Can you work these out from the model? Positions are in its coordinate system, mm. Face numbers are marked on the shaded views. A direction names the side the tool comes from. Coordinates: 2 decimals unless noted, no trailing zeros. Order: outer loops, then holes, each group sorted by start corner. A loop starts at its lowest first (then second) coordinate and runs counter-clockwise, first axis right, second up. Notation, with made-up numbers: (-36.75, 63) -> (20.25, 63) arc R27 cw to (20.25, 79) -> close; hole circle Ø7 at (19, 32). An arc over 180 degrees is marked (long way). Write item = value, one per line.
```python
from build123d import *

# Parameters (mm, degrees)
SKETCH_1_W          = 179
SKETCH_1_H          = 182
EXTRUDE_1_DEPTH     = 15
SKETCH_2_R          = 15
CUT_EXTRUDE_1_DEPTH = 129.51556326
CUT_EXTRUDE_3_DEPTH = 129.51556326
FILLET_1_R          = 20
EXTRUDE_2_DEPTH     = 90
FILLET_2_R          = 15
EXTRUDE_3_DEPTH     = 5
SKETCH_7_W          = 172
SKETCH_7_H          = 155
EXTRUDE_4_DEPTH     = 15
CUT_EXTRUDE_4_DEPTH = 15
FILLET_3_R          = 48
SKETCH_9_R          = 4.5
CUT_EXTRUDE_5_DEPTH = 15
SKETCH_11_W         = 69
SKETCH_11_H         = 3
EXTRUDE_5_DEPTH     = 18
FILLET_4_R          = 18
SKETCH_12_R         = 12
CUT_EXTRUDE_6_DEPTH = 12
SKETCH_13_R         = 11
CUT_EXTRUDE_7_DEPTH = 6
FILLET_5_R          = 2


with BuildPart() as part:
    # 草图1 → 凸台-拉伸1 (new body)
    with BuildSketch(Plane(origin=(0, 0, 0), x_dir=(1, 0, 0), z_dir=(0, 1, 0))):
        Rectangle(SKETCH_1_W, SKETCH_1_H)
    extrude(amount=EXTRUDE_1_DEPTH)

    # 草图2 → 切除-拉伸1 (cut, through all)
    with BuildSketch(Plane(origin=(0, 15, 0), x_dir=(1, 0, 0), z_dir=(0, 1, 0))):
        with Locations(Location((0, 22, 0), (0, 0, 270))):
            Circle(SKETCH_2_R)
    extrude(amount=-CUT_EXTRUDE_1_DEPTH, mode=Mode.SUBTRACT)

    # 草图4 → 切除-拉伸3 (cut, through all)
    with BuildSketch(Plane(origin=(0, 15, 0), x_dir=(1, 0, 0), z_dir=(0, 1, 0))):
        with BuildLine():
            Line((-77, -72.5), (-73, -72.5))
            ThreePointArc((-73, -72.5), (-67.5, -78), (-73, -83.5))
            Line((-73, -83.5), (-77, -83.5))
            ThreePointArc((-77, -83.5), (-82.5, -78), (-77, -72.5))
        make_face()
        with BuildLine():
            Line((-77, -22.5), (-73, -22.5))
            ThreePointArc((-73, -22.5), (-67.5, -28), (-73, -33.5))
            Line((-73, -33.5), (-77, -33.5))
            ThreePointArc((-77, -33.5), (-82.5, -28), (-77, -22.5))
        make_face()
        with BuildLine():
            Line((-77, 7.5), (-73, 7.5))
            ThreePointArc((-73, 7.5), (-67.5, 2), (-73, -3.5))
            Line((-73, -3.5), (-77, -3.5))
            ThreePointArc((-77, -3.5), (-82.5, 2), (-77, 7.5))
        make_face()
        with BuildLine():
            Line((77, 7.5), (73, 7.5))
            ThreePointArc((73, 7.5), (67.5, 2), (73, -3.5))
            Line((73, -3.5), (77, -3.5))
            ThreePointArc((77, -3.5), (82.5, 2), (77, 7.5))
        make_face()
        with BuildLine():
            Line((77, -22.5), (73, -22.5))
            ThreePointArc((73, -22.5), (67.5, -28), (73, -33.5))
            Line((73, -33.5), (77, -33.5))
            ThreePointArc((77, -33.5), (82.5, -28), (77, -22.5))
        make_face()
        with BuildLine():
            Line((77, -72.5), (73, -72.5))
            ThreePointArc((73, -72.5), (67.5, -78), (73, -83.5))
            Line((73, -83.5), (77, -83.5))
            ThreePointArc((77, -83.5), (82.5, -78), (77, -72.5))
        make_face()
    extrude(amount=-CUT_EXTRUDE_3_DEPTH, mode=Mode.SUBTRACT)

    # 圆角1
    fillet_1_edges = [part.edges().sort_by_distance(p)[0] for p in [
        (89.5, 7.5, 91),
        (-89.5, 7.5, 91),
    ]]
    fillet(fillet_1_edges, radius=FILLET_1_R)

    # 草图5 → 凸台-拉伸2 (add)
    with BuildSketch(Plane(origin=(0, 15, 0), x_dir=(1, 0, 0), z_dir=(0, 1, 0))):
        Polygon((-64, 91), (-64, -45), (64, -45), (64, 91), (39, 91), (39, -29), (-39, -29), (-39, 91), align=None)
    extrude(amount=EXTRUDE_2_DEPTH)

    # 圆角2
    fillet_2_edges = [part.edges().sort_by_distance(p)[0] for p in [
        (-64, 60, 45),
        (64, 60, 45),
    ]]
    fillet(fillet_2_edges, radius=FILLET_2_R)

    # 草图6 → 凸台-拉伸3 (add, symmetric)
    with BuildSketch(Plane(origin=(0, 0, 0), x_dir=(0, 0, -1), z_dir=(1, 0, 0))):
        with BuildLine():
            Line((-45, 105), (-60, 105))
            Line((-60, 105), (-49, 80))
            Line((-49, 80), (-49, 54.937451095))
            ThreePointArc((-49, 54.937451095), (-57.014709064, 30.259525737), (-78, 15))
            Line((-78, 15), (-45, 15))
            Line((-45, 15), (-45, 105))
        make_face()
    extrude(amount=EXTRUDE_3_DEPTH, both=True)

    # 草图7 → 凸台-拉伸4 (add)
    with BuildSketch(Plane(origin=(0, 105, 0), x_dir=(1, 0, 0), z_dir=(0, 1, 0))):
        with Locations((0, 13.5)):
            Rectangle(SKETCH_7_W, SKETCH_7_H)
    extrude(amount=EXTRUDE_4_DEPTH)

    # 草图8 → 切除-拉伸4 (cut)
    with BuildSketch(Plane(origin=(0, 120, 0), x_dir=(1, 0, 0), z_dir=(0, 1, 0))):
        Polygon((-86, 91), (-86, 60), (-64, 91), align=None)
        Polygon((64, 91), (86, 91), (86, 60), align=None)
    extrude(amount=-CUT_EXTRUDE_4_DEPTH, mode=Mode.SUBTRACT)

    # 圆角3
    fillet_3_edges = [part.edges().sort_by_distance(p)[0] for p in [
        (-86, 112.5, 64),
        (86, 112.5, 64),
    ]]
    fillet(fillet_3_edges, radius=FILLET_3_R)

    # 草图9 → 切除-拉伸5 (cut)
    with BuildSketch(Plane(origin=(0, 120, 0), x_dir=(1, 0, 0), z_dir=(0, 1, 0))):
        with Locations(Location((-72, 60, 0), (0, 0, 270))):
            Circle(SKETCH_9_R)
        with Locations(Location((-72, -16, 0), (0, 0, 270))):
            Circle(SKETCH_9_R)
        with Locations(Location((72, -16, 0), (0, 0, 270))):
            Circle(SKETCH_9_R)
        with Locations(Location((72, 60, 0), (0, 0, 270))):
            Circle(SKETCH_9_R)
    extrude(amount=-CUT_EXTRUDE_5_DEPTH, mode=Mode.SUBTRACT)

    # 草图11 → 凸台-拉伸5 (add, symmetric)
    with BuildSketch(Plane(origin=(0, 0, 0), x_dir=(0, 0, -1), z_dir=(1, 0, 0))):
        with Locations((5.5, 103.5)):
            Rectangle(SKETCH_11_W, SKETCH_11_H)
    extrude(amount=EXTRUDE_5_DEPTH, both=True)

    # 圆角4
    fillet_4_edges = [part.edges().sort_by_distance(p)[0] for p in [
        (-18, 103.5, -40),
        (18, 103.5, -40),
    ]]
    fillet(fillet_4_edges, radius=FILLET_4_R - 0.0001)  # a hair under: the kernel refuses the full size

    # 草图12 → 切除-拉伸6 (cut)
    with BuildSketch(Plane(origin=(0, 120, 0), x_dir=(1, 0, 0), z_dir=(0, 1, 0))):
        with Locations(Location((0, 22, 0), (0, 0, 270))):
            Circle(SKETCH_12_R)
    extrude(amount=-CUT_EXTRUDE_6_DEPTH, mode=Mode.SUBTRACT)

    # 草图13 → 切除-拉伸7 (cut)
    with BuildSketch(Plane(origin=(0, 108, 0), x_dir=(1, 0, 0), z_dir=(0, 1, 0))):
        with Locations(Location((0, 22, 0), (0, 0, 270))):
            Circle(SKETCH_13_R)
    extrude(amount=-CUT_EXTRUDE_7_DEPTH, mode=Mode.SUBTRACT)

    # 圆角5
    fillet_5_edges = [part.edges().sort_by_distance(p)[0] for p in [
        (-64, 15, -30.5),
        (64, 15, -30.5),
        (-27, 15, 45),
        (59.606601718, 15, 40.606601718),
        (-59.606601718, 15, 40.606601718),
        (27, 15, 45),
        (-5, 60, 45),
        (-5, 105, 52.5),
        (-5, 15, 61.5),
        (5, 60, 45),
        (5, 105, 52.5),
        (5, 15, 61.5),
    ]]
    fillet(fillet_5_edges, radius=FILLET_5_R)


solid = part.part
```
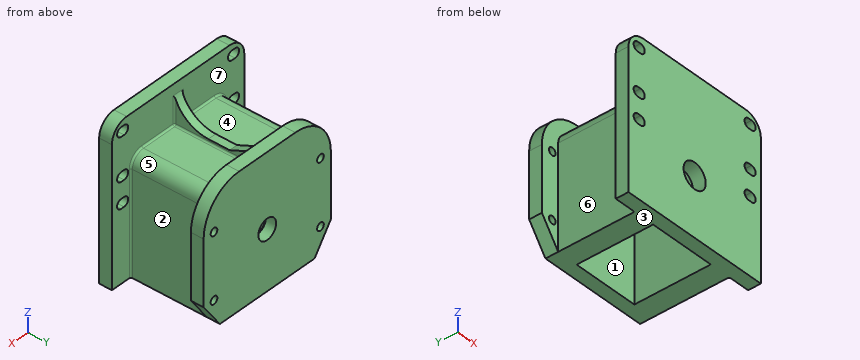
Item 1: If I drill on probe 1 along X at (y, z) = (113.5, -60); probe 2 along Y at (x, z) = (67, -11); probe 3 along X at (y, z) = (92.5, -34), over which ranges is the centre line in solid material (lowest first)?
A:
probe_1 = -86 to -76.5, -67.5 to 67.5, 76.5 to 86
probe_2 = 0 to 15, 105 to 120
probe_3 = -64 to -39, 39 to 64
Item 2: I want a section at D-D, the plane y = 33. Please give me the cut outline in (x, z), plus the area to 4 significant figures.
A:
outline = (-64, -91) -> (-39, -91) -> (-39, 29) -> (39, 29) -> (39, -91) -> (64, -91) -> (64, 30) arc R15 ccw to (49, 45) -> (7, 45) arc R2 cw to (5, 47) -> (5, 55.18) -> (-5, 55.18) -> (-5, 47) arc R2 cw to (-7, 45) -> (-49, 45) arc R15 ccw to (-64, 30) -> close
area = 8,055 mm2
Item 3: If we mould it in two halves opening along X, with no side actions, what happens to the marked faces 1, 2 and 3? For each: pulls with the +X half, pulls with the -X half, needs draft (parallel to the pull), parting line crosses it, or undercut.
A:
face_1 = undercut
face_2 = pulls with the +X half
face_3 = needs draft
Item 4: I'm going to push flat-ended pins straight in: P1, Ø1, axis at x = -11.5, y = 25.5, coming from the -Z side; P2, Ø2, axis at y = 92, z = -42.5, coming from the -X side; P3, Ø21, axis at x = -36.5, y = 61.5, coming from the +Z side. Where does each tip first touch, or does it pass through?
A:
P1 = 29
P2 = -64
P3 = 45
Item 5: For the marked faces 4, 5, 6 and 7, which set-ups out of +Z, -Z, +X, -X, +Y, -Y let a thin tool reach every point of the face, with its end or its side?
A:
face_4 = +Z, -X
face_5 = +Z, +X
face_6 = +Z, -Z, -X
face_7 = +Z
Item 6: I want a section at C-C, the plane z = 55.5. Please give me the cut outline in (x, y).
A:
outline = (-89.5, 0) -> (89.5, 0) -> (89.5, 15) -> (7, 15) arc R2 cw to (5, 17) -> (5, 32.49) -> (-5, 32.49) -> (-5, 17) arc R2 cw to (-7, 15) -> (-89.5, 15) -> close; (-65.27, 105) -> (-7, 105) arc R2 cw to (-5, 103) -> (-5, 94.77) -> (5, 94.77) -> (5, 103) arc R2 cw to (7, 105) -> (65.27, 105) -> (65.27, 120) -> (-65.27, 120) -> close
Item 7: I want a section at B-B, the plane x = -24. Please give me the cut outline in (y, z).
A:
outline = (0, -91) -> (15, -91) -> (15, 29) -> (105, 29) -> (105, -91) -> (120, -91) -> (120, 64) -> (105, 64) -> (105, 45) -> (17, 45) arc R2 cw to (15, 47) -> (15, 91) -> (0, 91) -> close
Item 8: I want a section at A-A, the plane y = 8. Give the number of separate pieces and of enclosed holes in the cut face, plus the area to 3 significant figures.
A:
separate_pieces = 1
enclosed_holes = 7
area = 30,900 mm2
